```python
from build123d import *

# Parameters (mm, degrees)
SKETCH1_R           = 76.2
SKETCH1_R_2         = 53.086
BOSS_EXTRUDE2_DEPTH = 6.35
CUT_EXTRUDE1_REACH  = 109.95
SKETCH2_W           = 12.7
SKETCH2_H           = 6.35
CIRPATTERN1_COUNT   = 4
BOSS_EXTRUDE3_START = -6.35
SKETCH3_R           = 53.086
BOSS_EXTRUDE3_DEPTH = 6.35


with BuildPart() as part:
    # Sketch1 → Boss-Extrude2 (new body)
    with BuildSketch(Plane.XY):
        Circle(SKETCH1_R)
        Circle(SKETCH1_R_2, mode=Mode.SUBTRACT)
    extrude(amount=BOSS_EXTRUDE2_DEPTH)

    # Sketch2 → Cut-Extrude1 (cut, up to next)
    with BuildSketch(Plane.XY.offset(6.35), mode=Mode.PRIVATE) as cut_extrude1_sk1:
        with Locations((0, 70.4215)):
            Rectangle(SKETCH2_W, SKETCH2_H)
    cut_extrude1_tool1 = extrude(cut_extrude1_sk1.sketch, amount=-CUT_EXTRUDE1_REACH, mode=Mode.PRIVATE) & part.part
    # Sketch2 → Cut-Extrude1 (cut, up to next)
    with BuildSketch(Plane.XY.offset(6.35), mode=Mode.PRIVATE) as cut_extrude1_sk2:
        with Locations((0, 58.8645)):
            Rectangle(SKETCH2_W, SKETCH2_H)
    cut_extrude1_tool2 = extrude(cut_extrude1_sk2.sketch, amount=-CUT_EXTRUDE1_REACH, mode=Mode.PRIVATE) & part.part
    cut_extrude1_1 = cut_extrude1_tool1.solids().sort_by_distance((0, 70.4215, 6.35))[0]
    add(cut_extrude1_1, mode=Mode.SUBTRACT)
    cut_extrude1_2 = cut_extrude1_tool2.solids().sort_by_distance((0, 58.8645, 6.35))[0]
    add(cut_extrude1_2, mode=Mode.SUBTRACT)
    cut_extrude1 = cut_extrude1_1 + cut_extrude1_2  # Cut-Extrude1 as one shape, for the pattern or mirror that repeats it

    # CirPattern1: Cut-Extrude1 ×4 about axis
    cirpattern1_axis = Axis((0, 0, 0), (0, 0, 1))
    for i in range(1, CIRPATTERN1_COUNT):
        add(cut_extrude1.rotate(cirpattern1_axis, i * 360 / CIRPATTERN1_COUNT), mode=Mode.SUBTRACT)

    # Sketch3 → Boss-Extrude3 (add)
    with BuildSketch(Plane.XY.offset(6.35).offset(BOSS_EXTRUDE3_START)):
        Circle(SKETCH3_R)
    extrude(amount=BOSS_EXTRUDE3_DEPTH)


solid = part.part
```
Read the model definition and answer for the solid it produces. Units are mm, in the model's axes. A direction names the side the tool comes from. Give positions to 0.01 mm unless a question says otherwise; leave off trailing zeros. Loops run counter-clockwise (first coordinate to the right, second up) from the corner with the lowest first, then second, coordinate; pieces in that order, holes last.
Item 1: The part is cut by section D-D (y = -57.5). Write down the section's boundary in (x, z).
Item 2: The part is cut by section B-B (x = 0). Write down the section's boundary in (y, z), and give its area (3 significant figures).
Item 3: The part is cut by section A-A (z = 1.75). Give the number of separate pieces and of enclosed holes in the cut face, and give its area (3 significant figures).
Item 4: The mould has two halves that part along Y. Classify faces 3 (the flat face through (67.246, 0, 3)), 4 (the flat face through (-1, 1, 6.35)), 5 (the flat face through (73.596, 0, 3)): released by +Y, released by -Y, zero draft, split by the parting line, or undercut.
Item 5: For faces 1 (the flat face through (-1, 1, 0)), 2 (the flat face through (0, -73.596, 3)), determine the directions among +Z, -Z, +X, -X, +Y, -Y from which every point of the face is accessible in a straight line to the end or side of a thin tool.
Item 6: Each of these flat-tipped pins is pushed along its axis until it touches: pin 1 Ø2 at (x, z) = (-30.5, 2.5) entering from +Y; pin 2 Ø1.9 at (y, z) = (0.5, 3.5) entering from +X; pin 3 Ø1.5 at (x, z) = (-30, 3) entering from +Y; pin 4 Ø3 at (x, z) = (69, 4.5) entering from -Y. Where does it stop, or does it pass through?
Item 7: Find the intervals of material crossed by line 1 along X through (y, z) = (61, 1.5); line 2 along Y through (x, z) = (-4.5, 3.5); line 3 along Y through (x, z) = (62, 1), in increasing order.
Taken from the geometry:
1. outline: (-50, 0) - (-6.35, 0) - (-6.35, 6.35) - (-50, 6.35) - close; (6.35, 0) - (50, 0) - (50, 6.35) - (6.35, 6.35) - close
2. outline: (-76.2, 0) - (-73.6, 0) - (-73.6, 6.35) - (-76.2, 6.35) - close; (-67.25, 0) - (-62.04, 0) - (-62.04, 6.35) - (-67.25, 6.35) - close; (-55.69, 0) - (55.69, 0) - (55.69, 6.35) - (-55.69, 6.35) - close; (62.04, 0) - (67.25, 0) - (67.25, 6.35) - (62.04, 6.35) - close; (73.6, 0) - (76.2, 0) - (76.2, 6.35) - (73.6, 6.35) - close
2. area: 806 mm2
3. separate pieces: 1
3. enclosed holes: 8
3. area: 17,600 mm2
4. face 3: undercut
4. face 4: zero draft
4. face 5: undercut
5. face 1: -Z, +X, -X, +Y, -Y
5. face 2: +Z, -Z
6. pin 1: stops at y = 70.26
6. pin 2: stops at x = 76.2
6. pin 3: stops at y = 70.36
6. pin 4: stops at y = -35.36
7. line 1: x = -45.67 to -6.35, 6.35 to 45.67
7. line 2: y = -76.07 to -73.6, -67.25 to -62.04, -55.69 to 55.69, 62.04 to 67.25, 73.6 to 76.07
7. line 3: y = -44.3 to -6.35, 6.35 to 44.3
